Geometry: final body of the model. Coordinates: model frame, mm. Face numbers are marked on the shaded views. A direction names the side the tool comes from. Give positions to 0.01 mm unless a question says otherwise; leave off trailing zeros. Write each loop counter-clockwise with the first axis right and the second up, starting at its lowest first coordinate (ties: lowest second). Pieces come first, ordered by that corner, then holes. Notation, with made-up numbers: (81.25, -39.75) - (136.25, -39.75) arc R17 ccw to (136.25, -24.75) - close; hole circle Ø8 at (53, 69.25). An arc over 180 degrees is marked (long way). Return JSON: item names as keys, results as strings.
from build123d import *

# Parameters (mm, degrees)
CROQUIS3_W              = 100
CROQUIS3_H              = 60
SALIENTE_EXTRUIR1_DEPTH = 5
CROQUIS3_3_W            = 10
CROQUIS3_3_H            = 60
SALIENTE_EXTRUIR2_DEPTH = 100
CROQUIS5_R              = 6
CORTAR_EXTRUIR1_DEPTH   = 20


with BuildPart() as part:
    # Croquis3 → Saliente-Extruir1 (new body)
    with BuildSketch(Plane.XY):
        Rectangle(CROQUIS3_W, CROQUIS3_H)
    extrude(amount=-SALIENTE_EXTRUIR1_DEPTH)

    # Croquis3<3> → Saliente-Extruir2 (add)
    with BuildSketch(Plane.XY):
        Rectangle(CROQUIS3_3_W, CROQUIS3_3_H)
    extrude(amount=SALIENTE_EXTRUIR2_DEPTH)

    # Croquis5 → Cortar-Extruir1 (cut)
    with BuildSketch(Plane(origin=(5, 0, 0), x_dir=(0, 0, -1), z_dir=(1, 0, 0))):
        with Locations((-75, 0)):
            Circle(CROQUIS5_R)
        with Locations((-25, 0)):
            Circle(CROQUIS5_R)
    extrude(amount=-CORTAR_EXTRUIR1_DEPTH, mode=Mode.SUBTRACT)


solid = part.part
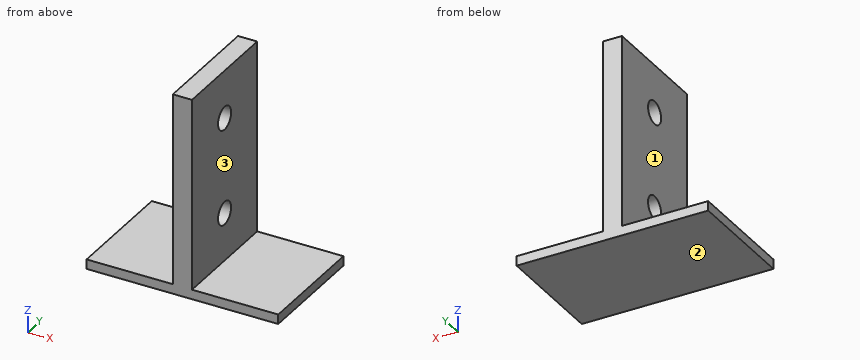
Q1. Section query C-C, the plane x = 2. Return the cut outline in (y, z).
Answer key:
{"outline": "(-30, -5) - (30, -5) - (30, 100) - (-30, 100) - close; hole circle Ø12 at (0, 25); hole circle Ø12 at (0, 75)"}
Q2. Set-up query: the marked faces 1, 2 and 3. Return all of +Z, -Z, +X, -X, +Y, -Y with unobstructed straight access to the full face (end or side cutting, diameter ignored); none if empty.
Answer key:
{"face 1": "+Z, -X, +Y, -Y", "face 2": "-Z, +X, -X, +Y, -Y", "face 3": "+Z, +X, +Y, -Y"}
Q3. Section query B-B, the plane y = 0. Return the cut outline in (x, z).
Answer key:
{"outline": "(-50, -5) - (50, -5) - (50, 0) - (5, 0) - (5, 19) - (-5, 19) - (-5, 0) - (-50, 0) - close; (-5, 31) - (5, 31) - (5, 69) - (-5, 69) - close; (-5, 81) - (5, 81) - (5, 100) - (-5, 100) - close"}
Q4. Section query D-D, the plane y = -14.5. Return the cut outline in (x, z).
Answer key:
{"outline": "(-50, -5) - (50, -5) - (50, 0) - (5, 0) - (5, 100) - (-5, 100) - (-5, 0) - (-50, 0) - close"}
Q5. Section query A-A, the plane z = 75. Return the cut outline in (x, y).
Answer key:
{"outline": "(-5, -30) - (5, -30) - (5, -6) - (-5, -6) - close; (-5, 6) - (5, 6) - (5, 30) - (-5, 30) - close"}
Q6. Pin query (flat end, axial travel): P1, Ø3, axis at y = -18.5, z = 81.5, coming from the +X side; P2, Ø11, axis at y = 0, z = 25, coming from the +X side; P3, Ø5, axis at x = -40, y = 21.5, coming from the +Z side. Return the tip coordinate at first contact, or that it passes through.
Answer key:
{"P1": "stops at x = 5", "P2": "passes through", "P3": "stops at z = 0"}
Q7. Material intervals for probe 1 along Y at (x, z) = (-0.25, 25); probe 2 along X at (y, z) = (9.5, 69); probe 3 along Z at (x, y) = (35.5, -1), sorted ascending. Write a range as [from, to].
Answer key:
{"probe 1": "y = [-30, -6], [6, 30]", "probe 2": "x = [-5, 5]", "probe 3": "z = [-5, 0]"}
